from build123d import *

# Parameters (mm, degrees)
SHAPEBINDER_R = 2.8
PAD_DEPTH     = 5


with BuildPart() as part:
    # ShapeBinder → Pad (new body)
    with BuildSketch(Plane(origin=(65, 42.5, 0), x_dir=(0, -1, 0), z_dir=(0, 0, -1))):
        with BuildLine():
            Line((35, 65), (-35, 65))
            ThreePointArc((-35, 65), (-40.303301, 62.803301), (-42.5, 57.5))
            Line((-42.5, 57.5), (-42.5, -57.5))
            ThreePointArc((-42.5, -57.5), (-40.303301, -62.803301), (-35, -65))
            Line((-35, -65), (0.97016, -65))
            Line((0.97016, -65), (16.010767, -65))
            Line((16.010767, -65), (35, -65))
            ThreePointArc((35, -65), (40.303301, -62.803301), (42.5, -57.5))
            Line((42.5, -57.5), (42.5, 57.5))
            ThreePointArc((42.5, 57.5), (40.303301, 62.803301), (35, 65))
        make_face()
        with Locations((35.866117, 58.366117)):
            Circle(SHAPEBINDER_R, mode=Mode.SUBTRACT)
        with Locations((35.866117, -58.366117)):
            Circle(SHAPEBINDER_R, mode=Mode.SUBTRACT)
        with Locations((-35.866117, 58.366117)):
            Circle(SHAPEBINDER_R, mode=Mode.SUBTRACT)
        with BuildLine():
            ThreePointArc((28.639867, 59.333333), (31.428932, 53.928932), (36.833333, 51.139867))
            ThreePointArc((36.833333, 51.139867), (38.027525, 50.458835), (38.5, 49.16784))
            Line((38.5, 49.16784), (38.5, -49.16784))
            ThreePointArc((38.5, -49.16784), (38.027525, -50.458835), (36.833333, -51.139867))
            ThreePointArc((36.833333, -51.139867), (31.428932, -53.928932), (28.639867, -59.333333))
            ThreePointArc((28.639867, -59.333333), (27.958835, -60.527525), (26.66784, -61))
            Line((26.66784, -61), (-26.66784, -61))
            ThreePointArc((-26.66784, -61), (-27.958835, -60.527525), (-28.639867, -59.333333))
            ThreePointArc((-28.639867, -59.333333), (-31.428932, -53.928932), (-36.833333, -51.139867))
            ThreePointArc((-36.833333, -51.139867), (-38.027525, -50.458835), (-38.5, -49.16784))
            Line((-38.5, -49.16784), (-38.5, 49.16784))
            ThreePointArc((-38.5, 49.16784), (-38.027525, 50.458835), (-36.833333, 51.139867))
            ThreePointArc((-36.833333, 51.139867), (-31.428932, 53.928932), (-28.639867, 59.333333))
            ThreePointArc((-28.639867, 59.333333), (-27.958835, 60.527525), (-26.66784, 61))
            Line((-26.66784, 61), (26.66784, 61))
            ThreePointArc((26.66784, 61), (27.958835, 60.527525), (28.639867, 59.333333))
        make_face(mode=Mode.SUBTRACT)
        with Locations((-35.866117, -58.366117)):
            Circle(SHAPEBINDER_R, mode=Mode.SUBTRACT)
    extrude(amount=PAD_DEPTH)


solid = part.part
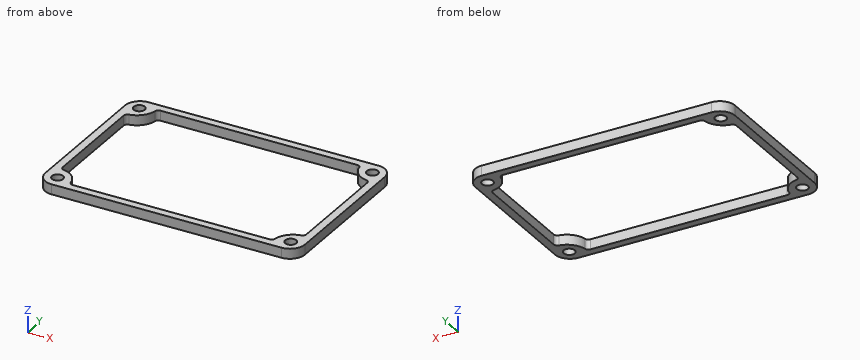
Build history of the part. All positions in model axes, mm. Round coordinates to 2 decimals unless told otherwise and drop trailing zeros. Loops run counter-clockwise (first coordinate to the right, second up) from the corner with the lowest first, then second, coordinate; pieces in that order, holes last. Notation, with made-up numbers: (77.25, -28.5) -> (112.25, -28.5) arc R25 ccw to (112.25, 10.5) -> close; hole circle Ø6 at (80, 19). An arc over 180 degrees is marked (long way). Use CSV: the item, a comma, the result in double quotes. Start each with the question number.
Q1. Drill centre lines: L1, parallel to Y at x = 79.5, z = -3.5; L2, parallel to X at y = 8, z = -4.5; L3, parallel to X at y = 47.5, z = -1.75. Where is each one in solid material? Low to high.
Q2. Saw through at A-A on y = 44.5. Give the cut face in (x, z), and give its area (3 significant figures).
Q3. Saw through at B-B on x = 77.5. Give the cut face in (y, z).
Q4. Saw through at C-C on z = -0.75. Give the cut face in (x, y), and give its area (3 significant figures).
Solutions:
1,L1,"y = 0 to 4, 81 to 85"
1,L2,"x = 0 to 4.19, 9.08 to 13.17, 116.83 to 120.92, 125.81 to 130"
1,L3,"x = 0 to 4, 126 to 130"
2,outline,"(0, -5) -> (4, -5) -> (4, 0) -> (0, 0) -> close; (126, -5) -> (130, -5) -> (130, 0) -> (126, 0) -> close"
2,area,"40.0 mm^2"
3,outline,"(0, -5) -> (4, -5) -> (4, 0) -> (0, 0) -> close; (81, -5) -> (85, -5) -> (85, 0) -> (81, 0) -> close"
4,outline,"(0, 7.5) arc R7.5 ccw to (7.5, 0) -> (122.5, 0) arc R7.5 ccw to (130, 7.5) -> (130, 77.5) arc R7.5 ccw to (122.5, 85) -> (7.5, 85) arc R7.5 ccw to (0, 77.5) -> close; hole circle Ø5.6 at (6.63, 6.63); hole circle Ø5.6 at (6.63, 78.37); hole (4, 15.83) arc R2 ccw to (5.67, 13.86) arc R10 cw to (13.86, 5.67) arc R2 ccw to (15.83, 4) -> (114.17, 4) arc R2 ccw to (116.14, 5.67) arc R10 cw to (124.33, 13.86) arc R2 ccw to (126, 15.83) -> (126, 69.17) arc R2 ccw to (124.33, 71.14) arc R10 cw to (116.14, 79.33) arc R2 ccw to (114.17, 81) -> (15.83, 81) arc R2 ccw to (13.86, 79.33) arc R10 cw to (5.67, 71.14) arc R2 ccw to (4, 69.17) -> close; hole circle Ø5.6 at (123.37, 6.63); hole circle Ø5.6 at (123.37, 78.37)"
4,area,"1,830 mm^2"
